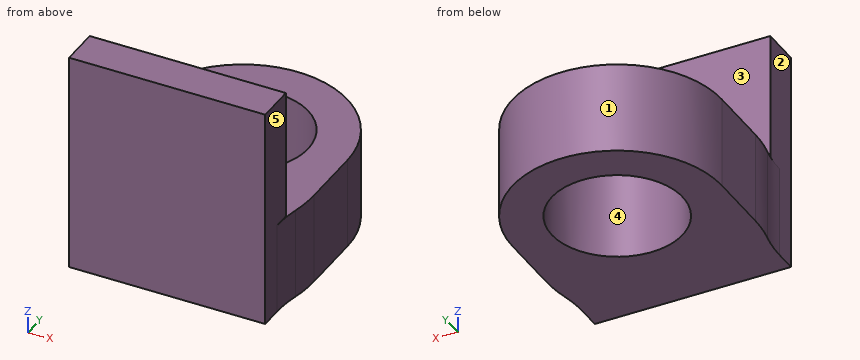
from build123d import *

# Parameters (mm, degrees)
SKETCH1_R           = 5
BOSS_EXTRUDE1_DEPTH = 7
SKETCH2_W           = 15
SKETCH2_H           = 3
BOSS_EXTRUDE2_DEPTH = 10
FILLET1_R           = 10
FILLET2_R           = 10


with BuildPart() as part:
    # Sketch1 → Boss-Extrude1 (new body)
    with BuildSketch(Plane.XY):
        with BuildLine():
            Line((-8, 0), (-8, -8))
            Line((-8, -8), (-7.5, -8))
            Line((-7.5, -8), (-7.5, -11))
            Line((-7.5, -11), (7.5, -11))
            Line((7.5, -11), (7.5, -8))
            Line((7.5, -8), (8, -8))
            Line((8, -8), (8, 0))
            ThreePointArc((8, 0), (0, 8), (-8, 0))
        make_face()
        Circle(SKETCH1_R, mode=Mode.SUBTRACT)
    extrude(amount=BOSS_EXTRUDE1_DEPTH)

    # Sketch2 → Boss-Extrude2 (add)
    with BuildSketch(Plane.XY.offset(7)):
        with Locations((0, -9.5)):
            Rectangle(SKETCH2_W, SKETCH2_H)
    extrude(amount=BOSS_EXTRUDE2_DEPTH)

    # Fillet1
    # the kernel refuses this fillet: 10 mm, written as the material it takes off along each edge
    with BuildSketch(Plane(origin=(-8, -8, -7.806247498), x_dir=(0, 1, 0), z_dir=(0, 0, 1))) as fillet1_piece_1:
        with BuildLine():
            CenterArc((3.122498999, -10), FILLET1_R, 90, 18.194872339)
            Line((0, -0.5), (0, 0))
            Line((0, 0), (3.122498999, 0))
        make_face()
    extrude(amount=22.612494996, mode=Mode.SUBTRACT)
    with BuildSketch(Plane(origin=(8, -8, -7.806247498), x_dir=(-1.0, 2.199129767162818e-12, 0), z_dir=(0, 0, 1))) as fillet1_piece_2:
        with BuildLine():
            CenterArc((10, -3.122498999), FILLET1_R, 161.805127661, 18.194872339)
            Line((0, -3.122498999), (0, 0))
            Line((0, 0), (0.5, 0))
        make_face()
    extrude(amount=22.612494996, mode=Mode.SUBTRACT)

    # Fillet2
    fillet2_edges = [part.edges().sort_by_distance(p)[0] for p in [
        (7.5, -8, 3.5),
        (-7.5, -8, 3.5),
    ]]
    fillet(fillet2_edges, radius=FILLET2_R)


solid = part.part
Geometry check sheet. Reference: the model listing, model coordinates, mm. Face numbers are marked on the shaded views. A direction names the side the tool comes from. Give positions to 0.01 mm unless a question says otherwise; leave off trailing zeros. Order: outer loops, then holes, each group sorted by start corner. A loop starts at its lowest first (then second) coordinate and runs counter-clockwise, first axis right, second up.
1) Cross-section at C-C (z = 15). Record the boundary of the cut face in (x, y), then the cut area to 3 significant figures.
Results are:
outline: (-7.5, -11) - (7.5, -11) - (7.5, -8) - (-7.5, -8) - close
area: 45.0 mm2
2) Gauge pin test, flat ends, axial feed: pin 1 (8 mm diameter, centred on x = 6, z = 5.5, fed in from +Y); pin 2 (3 mm diameter, centred on x = 2, z = 10.5, fed in from +Y); pin 3 (9 mm diameter, centred on x = 0, y = 0, fed in from +Z); pin 4 (3 mm diameter, centred on y = -7, z = 12.5, fed in from +X). Record the tip position at first contact, or that the pin passes through.
Results are:
pin 1: stops at y = 7.75
pin 2: stops at y = -8
pin 3: passes through
pin 4: stops at x = 7.5
3) Cross-section at D-D (y = -8.25). Record the boundary of the cut face in (x, z), then the cut area to 3 significant figures.
Results are:
outline: (-7.56, 0) - (7.56, 0) - (7.56, 7) - (7.5, 7) - (7.5, 17) - (-7.5, 17) - (-7.5, 7) - (-7.56, 7) - close
area: 256 mm2
4) Draft check along Y on the marked faces 3, 4 and 5. Enter one of: released by +Y, released by -Y, zero draft, split by the parting line, or undercut.
Results are:
face 3: released by +Y
face 4: undercut
face 5: zero draft
5) Tool access check on the marked faces 1 and 2. Record the directions out of +Z, -Z, +X, -X, +Y, -Y that give a thin tool (end or side, any length) a straight path to the whole face; none if there is none.
Results are:
face 1: +Z, -Z, +Y
face 2: +Z, -X, -Y
6) Cross-section at B-B (y = -0.75). Record the boundary of the cut face in (x, z), then the cut area to 3 significant figures.
Results are:
outline: (-8, 0) - (-4.94, 0) - (-4.94, 7) - (-8, 7) - close; (4.94, 0) - (8, 0) - (8, 7) - (4.94, 7) - close
area: 42.8 mm2
7) Material ranges on probe 1 along Y at (x, z) = (0, 5); probe 2 along Y at (x, z) = (-7, 9); probe 3 along X at (y, z) = (2.25, 4), recorded low to high.
Results are:
probe 1: y = -11 to -5, 5 to 8
probe 2: y = -11 to -8
probe 3: x = -7.68 to -4.47, 4.47 to 7.68
8) Cross-section at A-A (x = 0). Record the boundary of the cut face in (y, z).
Results are:
outline: (-11, 0) - (-5, 0) - (-5, 7) - (-8, 7) - (-8, 17) - (-11, 17) - close; (5, 0) - (8, 0) - (8, 7) - (5, 7) - close
